Verification items for the finished model (mm, model axes). A direction names the side the tool comes from. Coordinates: 2 decimals unless noted, no trailing zeros. Loops run counter-clockwise (first coordinate to the right, second up) from the corner with the lowest first, then second, coordinate; pieces in that order, holes last. Notation, with made-up numbers: (71.5, -23.5) - (92.5, -23.5) arc R6 ccw to (92.5, -12.5) - close; hole circle Ø6 at (84.25, -11.75). An arc over 180 degrees is marked (long way). Answer as CSV lines item,"result". Start each with the question number.
1. Set-up check for faces 4 (the flat face through (14, 4, -7)), 5 (the cylindrical face through (-12.07, 15.5, -16.52)), 6 (the flat face through (-2, 9, -11)): record each of +Z, -Z, +X, -X, +Y, -Y from which the full face is reachable in a straight line by a thin tool's end or side.
2. Cross-section at D-D (z = -14.25). Enter the section's corners in (x, y).
3. Material ranges on line 1 (Y direction, x = 0, z = -16.4); line 2 (Z direction, x = 11, y = 1); line 3 (X direction, y = 14, z = -17), recorded low to high. Write a range as [from, to].
4. Cross-section at C-C (y = 30). Enter the section's corners in (x, z).
5. Gauge pin test, flat ends, axial feed: P1, Ø4, axis at x = -11, z = -8, coming from the +Y side; P2, Ø5, axis at x = 12, y = 14, coming from the -Z side; P3, Ø7.5, axis at y = 14, z = -9.5, coming from the -X side; P4, Ø7.5, axis at y = 9.5, z = -8, coming from the +X side. Record the tip position at first contact, or that the pin passes through.
6. Cross-section at A-A (x = 0). Enter the section's corners in (y, z).
7. Release check for a two-part mould opening along X. For faces 1 (the flat face through (-5, 17, -15)), 2 (the cylindrical face through (11.9, 2, -9.2)), 3 (the cylindrical face through (8.578, 37.394, -16.521)) record: pulls with the +X half, pulls with the -X half, needs draft (parallel to the pull), parting line crosses it, or undercut.
8. Cross-section at B-B (z = -16.75). Enter the section's corners in (x, y).
Autodesk Inventor part; units mm, degrees
ref_plane "YZ Plane" through (0, 0, 0) normal (1, 0, 0) x (0, 1, 0)
ref_plane "XZ Plane" through (0, 0, 0) normal (0, 1, 0) x (-1, 0, 0)
ref_plane "XY Plane" through (0, 0, 0) normal (0, 0, 1) x (1, 0, 0)
sketch "Szkic1" plane through (0, 0, 0) normal (0, 1, 0) x (-1, 0, 0)
  line L0 (25, 19) -> (-25, 19)
  line L1 (-25, 19) -> (-25, -19)
  line L2 (-25, -19) -> (25, -19)
  line L3 (25, -19) -> (25, 19)
  line L4 (25, 19) -> (-25, -19) construction
  line L5 (-25, 19) -> (25, -19) construction
  point P0 (0, 0)
  dimension "d0" = 50
  dimension "d1" = 38
extrude "Wyciągnięcie proste1" add sketch "Szkic1" along normal blind 4
sketch "Szkic2" plane through (0, 4, 0) normal (0, 1, 0) x (1, 0, 0)
  line L0 (-25, 19) -> (-25, -19)
  line L1 (25, -19) -> (25, 19)
  line L2 (-25, 19) -> (25, 19)
  line L3 (25, 19) -> (25, 15)
  line L4 (25, 15) -> (-25, 15)
  line L5 (-25, 15) -> (-25, 19)
  point P0 (0, 0)
  dimension "d4" = 4
extrude "Wyciągnięcie proste2" add sketch "Szkic2" along normal blind 34
sketch "Szkic3" plane through (0, 4, 0) normal (0, 1, 0) x (1, 0, 0)
  line L0 (25, -19) -> (25, 19)
  line L1 (25, 0) -> (-25, 0) construction
  line L2 (-25, 19) -> (-25, -19)
  line L3 (-25, 15) -> (25, 15)
  line L4 (0, 15) -> (0, -19) construction
  line L5 (0, -15) -> (0, 19) construction
  point P0 (0, 0)
  point P1 (-11, 8)
  point P2 (-11, -8)
  point P3 (11, 8)
  point P4 (11, -8)
  dimension "d7" = 8
  dimension "d8" = 11
hole "Otwór1" at (-11, 4, -8) at (-11, 4, 8) at (11, 4, 8) at (11, 4, -8) direction (0, -1, 0) diameter 3 depth 8 tip angle 118
sketch "Szkic4" plane through (-25, 4, -15) normal (0, 0, 1) x (1, 0, 0)
  line L0 (50, 34) -> (0, 34)
  line L1 (0, 0) -> (0, 34)
  line L2 (50, 0) -> (0, 0)
  line L3 (25, 34) -> (25, 0) construction
  point P0 (25, -4)
  point P1 (25, 26)
  point P2 (13, 10)
  point P3 (37, 10)
  dimension "d16" = 8
  dimension "d17" = 25
  dimension "d18" = 13
  dimension "d19" = 10
hole "Otwór2" at (0, 30, -15) at (-12, 14, -15) at (12, 14, -15) direction (0, 0, -1) diameter 3 depth 8 tip angle 118
sketch "Szkic5" plane through (-25, 4, -15) normal (0, 0, 1) x (1, 0, 0)
  line L0 (0, 34) -> (50, 34)
  line L1 (50, 0) -> (50, 34)
  line L2 (50, 0) -> (0, 0)
  line L3 (34, 34) -> (50, 0)
  line L4 (34, 34) -> (50, 34)
  line L5 (50, 34) -> (50, 0)
  line L6 (25, 34) -> (25, 0) construction
  line L7 (50, 34) -> (0, 34)
  line L8 (0, 0) -> (0, 34)
  line L9 (0, 0) -> (50, 0)
  line L10 (16, 34) -> (0, 0)
  line L11 (16, 34) -> (0, 34)
  line L12 (0, 34) -> (0, 0)
  point P0 (25, -4)
  dimension "d27" = 16
extrude "Wyciągnięcie proste3" cut sketch "Szkic5" against normal blind 34 contours L0 L10 L8 | L0 L1 L3
fillet "Zaokrąglenie1" radius 4 2 edges at (-9, 38, -17) (9, 38, -17)
sketch "Szkic9" plane through (25, 0, 19) normal (1, 0, 0) x (0, 0, -1)
  line L0 (38, 0) -> (0, 0)
  line L1 (38, 0) -> (37, 0)
  line L2 (37, 0) -> (37, 38)
  line L3 (37, 38) -> (38, 38)
  line L4 (38, 38) -> (38, 0)
  point P0 (19, 0)
  dimension "d38" = 1
  dimension "d39" = 38
extrude "Wyciągnięcie proste6" cut sketch "Szkic9" against normal through all
sketch "Szkic10" plane through (0, 0, 0) normal (0, -1, 0) x (1, 0, 0)
  line L0 (25, 19) -> (25, -15)
  line L1 (-25, -15) -> (-25, 19)
  line L2 (25, 19) -> (-25, 19)
  line L3 (-25, 19) -> (-25, 0)
  line L4 (-25, 0) -> (25, 0)
  line L5 (25, 0) -> (25, 19)
  point P0 (0, 0)
  dimension "d42" = 19
extrude "Wyciągnięcie proste7" cut sketch "Szkic10" against normal blind 10
sketch "Szkic11" plane through (0, 4, 0) normal (0, 1, 0) x (1, 0, 0)
  line L0 (25, 0) -> (-25, 0)
  line L1 (-6.4616, 15) -> (6.4616, 15)
  line L2 (2, 0) -> (-2, 0)
  line L3 (-2, 0) -> (-2, 15)
  line L4 (-2, 15) -> (2, 15)
  line L5 (2, 15) -> (2, 0)
  point P0 (0, 0)
  dimension "d45" = 4
  dimension "d46" = 2
extrude "Wyciągnięcie proste8" add sketch "Szkic11" along normal blind 20
sketch "Szkic12" plane through (2, 4, 0) normal (1, 0, 0) x (0, 0, -1)
  line L0 (15, 20) -> (15, 0)
  line L1 (15, 20) -> (0, 0)
  line L2 (0, 0) -> (0, 20)
  line L3 (0, 0) -> (0, 20)
  line L4 (15, 20) -> (0, 20)
  line L5 (0, 20) -> (15, 20)
  point P0 (0, -4)
extrude "Wyciągnięcie proste9" cut sketch "Szkic12" against normal blind 20
chamfer "Faza1" distance 10 angle 45 2 edges at (25, 2, 0) (-25, 2, 0)
properties part number "Wspornik_góra" material "Tworzywo sztuczne PET"
Values follow:
1,face 4,"+Z, +X, +Y"
1,face 5,"+Z, -Z"
1,face 6,"+Z, -X, +Y"
2,outline,"(-25, 0) - (25, 0) - (25, 4) - (2, 4) - (2, 23) - (-2, 23) - (-2, 4) - (-25, 4) - close"
3,line 1,"y = [0, 28.5], [31.5, 38]"
3,line 2,"z = [-18, -9.5], [-6.5, 0]"
3,line 3,"x = [-20.29, -13.5], [-10.5, 10.5], [13.5, 20.29]"
4,outline,"(-12.76, -18) - (-1.5, -18) - (-1.5, -15) - (-12.76, -15) - close; (1.5, -18) - (12.76, -18) - (12.76, -15) - (1.5, -15) - close"
5,P1,"stops at y = 4"
5,P2,"stops at z = -18"
5,P3,"stops at x = -2"
5,P4,"stops at x = 2"
6,outline,"(0, -18) - (28.5, -18) - (28.5, -15) - (24, -15) - (4, 0) - (0, 0) - close; (31.5, -18) - (38, -18) - (38, -15) - (31.5, -15) - close"
7,face 1,"needs draft"
7,face 2,"undercut"
7,face 3,"pulls with the +X half"
8,outline,"(-25, 0) - (25, 0) - (25, 4) - (10.08, 35.7) arc R4 ccw to (6.46, 38) - (-6.46, 38) arc R4 ccw to (-10.08, 35.7) - (-25, 4) - close; hole circle Ø3 at (-12, 14); hole circle Ø3 at (0, 30); hole circle Ø3 at (12, 14)"
